```python
from build123d import *

# Parameters (mm, degrees)
BOSS_EXTRUDE1_DEPTH = 2133.6
CUT_EXTRUDE2_DEPTH  = 613.218203925
SHELL1_T            = -7.9375


with BuildPart() as part:
    # Sketch1 → Boss-Extrude1 (new body)
    with BuildSketch(Plane.XY):
        Polygon((0, 0), (508, 0), (660.4, 406.4), (-152.4, 406.4), align=None)
    extrude(amount=BOSS_EXTRUDE1_DEPTH)

    # Sketch13 → Cut-Extrude2 (cut, symmetric, along a direction that is not the sketch's normal)
    with BuildSketch(Plane(origin=(254, 0, 0), x_dir=(0, 0, -1), z_dir=(1, 0, 0))):
        Polygon((-2133.6, 0), (-3174.648587482, 0), (-3174.648587482, 406.4), (-2133.6, 406.4), (-1676.4, 0), align=None)
    cut_extrude2 = extrude(amount=CUT_EXTRUDE2_DEPTH, dir=(0.664363839, 0, 0.747409319), both=True, mode=Mode.SUBTRACT)

    # Mirror1: Cut-Extrude2 across plane
    add(cut_extrude2.mirror(Plane(origin=(254, 0, 0), x_dir=(0, 0, 1), z_dir=(1, 0, 0))), mode=Mode.SUBTRACT)

    # Shell1
    shell1_openings = [part.faces().sort_by_distance(p)[0] for p in [
        (254, 406.4, 1097.28),
    ]]
    offset(amount=SHELL1_T, openings=shell1_openings, kind=Kind.INTERSECTION)


solid = part.part
```
The model under review builds one solid part; all positions refer to its coordinate system, in mm. A direction names the side the tool comes from. Round coordinates to 2 decimals unless told otherwise and drop trailing zeros. Write each loop counter-clockwise with the first axis right and the second up, starting at its lowest first coordinate (ties: lowest second). Pieces come first, ordered by that corner, then holes. Notation, with made-up numbers: (-5, 54.25) -> (48, 54.25) arc R22 cw to (48, 76.25) -> close; hole circle Ø7 at (78.5, 67.5). An arc over 180 degrees is marked (long way). Use CSV: the item, a comma, the result in double quotes.
Q1. To check wall thickness, follow probe 1 along X at (y, z) = (218.5, 1208); probe 2 along X at (y, z) = (111.5, 659); probe 3 along Z at (x, y) = (127, 183). State the ranges of each line that lie inside material, in increasing order. Write a range as [from, to].
Checks:
probe 1,"[-81.94, -73.46], [581.46, 589.94]"
probe 2,"[-41.81, -33.34], [541.34, 549.81]"
probe 3,"[0, 7.94], [1724.48, 1739.4]"
Q2. Consider section D-D (y = 272). Give the boundary of the cut face in (x, z), then the cut area to 3 significant figures.
Checks:
outline,"(-102, 0) -> (610, 0) -> (610, 1581.9) -> (254, 1982.4) -> (-102, 1581.9) -> close; hole (-93.52, 7.94) -> (601.52, 7.94) -> (601.52, 1576.52) -> (254, 1967.48) -> (-93.52, 1576.52) -> close"
area,"42,800 mm²"
Q3. For faces 4 (the flat face through (98.8, 222.79, 1752.44)), 5 (the flat face through (405.96, 226.41, 1745.24)), list the 3-axis set-ups (+Z, -Z, +X, -X, +Y, -Y) from which the entire face can be reached by the end or side of a thin tool; tool diameter is ignored.
Checks:
face 4,"+Z, -X, -Y"
face 5,"+Y"
Q4. For pin 1 Ø1.5 at (x, z) = (319, 1187) entering from -Y; pin 2 Ø1 at (y, z) = (77, 1349) entering from -X; pin 3 Ø10 at (y, z) = (281.5, 713) entering from -X; pin 4 Ø10 at (x, z) = (136, 1509) entering from +Y, all flat-tipped, find the tip position at first contact; note any pin that passes through.
Checks:
pin 1,"y = 0"
pin 2,"x = -29.06"
pin 3,"x = -107.44"
pin 4,"y = 7.94"
Q5. Consider section C-C (x = 587.5). Give the boundary of the cut face in (y, z).
Checks:
outline,"(212, 0) -> (406.4, 0) -> (406.4, 7.94) -> (234.61, 7.94) -> (234.61, 1550.23) -> (406.4, 1743.5) -> (406.4, 1758.41) -> (212, 1539.71) -> close"
Q6. Consider section B-B (y = 40). Give the boundary of the cut face in (x, z) (1 decimal), then the cut area to 3 significant figures.
Checks:
outline,"(-15, 0) -> (523, 0) -> (523, 1418.8) -> (254, 1721.4) -> (-15, 1418.8) -> close; hole (-6.5, 7.9) -> (514.5, 7.9) -> (514.5, 1413.4) -> (254, 1706.5) -> (-6.5, 1413.4) -> close"
area,"36,000 mm²"
Q7. Consider section A-A (z = 746). Give the boundary of the cut face in (x, y).
Checks:
outline,"(-152.4, 406.4) -> (0, 0) -> (508, 0) -> (660.4, 406.4) -> (651.92, 406.4) -> (502.5, 7.94) -> (5.5, 7.94) -> (-143.92, 406.4) -> close"
Q8. Mouldability with a two-part tool opening along X and no side actions: class faces 1 (the flat face through (-70.257, 209.958, 827.838)), 2 (the flat face through (409.2, 222.79, 1752.44)), 3 (the flat face through (-77.267, 206.045, 826.465)) as released by +X, released by -X, zero draft, split by the parting line, or undercut.
Checks:
face 1,"undercut"
face 2,"released by +X"
face 3,"released by -X"
